Could you check a few things on this model? Use its own coordinates, in mm. Face numbers are marked on the shaded views. A direction names the side the tool comes from. Give positions to 0.01 mm unless a question says otherwise; leave off trailing zeros. Loops run counter-clockwise (first coordinate to the right, second up) from the corner with the lowest first, then second, coordinate; pieces in that order, holes last. Notation, with made-up numbers: M 76.5,52.25 L 96.5,52.25 A18 ccw 96.5,81.25 Z; hole C 17,57.5 d9. An arc over 180 degrees is marked long. Return JSON: item names as keys, results as strings. Group by question number.
1. If we section it at D-D (z = 0.25): Write out the boundary of the cut face in (x, y).
2. For the marked faces 1, 2 and 3, which set-ups out of +Z, -Z, +X, -X, +Y, -Y let a thin tool reach every point of the face, with its end or its side?
3. If we mould it in two halves opening along Y, with no side actions, what happens to the marked faces 4, 5 and 6? For each: +Y half, -Y half, draft (parallel to the pull), parting line (faces both ways), or undercut.
4. If we section it at B-B (z = -6.25): Write out the boundary of the cut face in (x, y), plus the area to 3 significant figures.
5. Please list where these lines run through material, in increasing order: line 1 (X direction, y = -124, z = 0.25); line 2 (X direction, y = -98.5, z = -7.35); line 3 (Y direction, x = 53, z = 0.6).
6. If we section it at A-A (y = -98.5): Write out the boundary of the cut face in (x, z), plus the area to 3 significant figures.
7. For pin 1 (4.5 mm diameter, centred on x = 53, y = -98.5, fed in from +Z); pin 2 (11.5 mm diameter, centred on x = 51.5, y = -96.5, fed in from +Z); pin 3 (5.5 mm diameter, centred on x = 53, y = -132, fed in from +Z); pin 4 (14.5 mm diameter, centred on x = 52, y = -126.5, fed in from -Z), each with a flat end and sliding along its axis, tell me the tip position at first contact or that it passes through.
8. If we section it at C-C (y = -124): Write out the boundary of the cut face in (x, z).
```python
from build123d import *

# Parameters (mm, degrees)
PAD024_DEPTH    = 13.5
SKETCH067_R     = 2.9
POCKET045_DEPTH = 5.001
SKETCH068_R     = 5.5
POCKET046_DEPTH = 3
SKETCH069_R     = 2.1
POCKET047_DEPTH = 7.001
CHAMFER023_SIZE = 4.99
FILLET014_R     = 10
CHAMFER024_SIZE = 3
CHAMFER025_SIZE = 0.2
CHAMFER026_SIZE = 1
CHAMFER027_SIZE = 1
CHAMFER028_SIZE = 0.4


with BuildPart() as part:
    # Sketch066 → Pad024 (new body, symmetric)
    with BuildSketch(Plane.YZ):
        Polygon((23, 0), (0, 0), (0, 7), (-28, 7), (-28, 0), (-10, 0), (-10, -5), (23, -5), align=None)
    extrude(amount=PAD024_DEPTH, both=True)

    # Sketch067 → Pocket045 (cut, through all)
    with BuildSketch(Plane.XY):
        with Locations((0, 11.5)):
            Circle(SKETCH067_R)
    extrude(amount=-POCKET045_DEPTH, mode=Mode.SUBTRACT)

    # Sketch068 (on Face7 of Pocket045) → Pocket046 (cut)
    with BuildSketch(Plane(origin=(0, 0, -5), x_dir=(1, 0, 0), z_dir=(0, 0, -1))):
        with Locations((0, -11.5)):
            Circle(SKETCH068_R)
    extrude(amount=-POCKET046_DEPTH, mode=Mode.SUBTRACT)

    # Sketch069 (on Face10 of Pocket046) → Pocket047 (cut, through all)
    with BuildSketch(Plane(origin=(0, 0, 0), x_dir=(1, 0, 0), z_dir=(0, 0, -1))):
        with Locations((0, 22)):
            Circle(SKETCH069_R)
        with Locations((-6, 14)):
            Circle(SKETCH069_R)
        with Locations((6, 14)):
            Circle(SKETCH069_R)
    extrude(amount=-POCKET047_DEPTH, mode=Mode.SUBTRACT)

    # Chamfer023
    chamfer023_edges = [part.edges().sort_by_distance(p)[0] for p in [
        (0, -10, -5),
    ]]
    chamfer(chamfer023_edges, length=CHAMFER023_SIZE)

    # Fillet014
    fillet014_edges = [part.edges().sort_by_distance(p)[0] for p in [
        (13.5, 23, -2.5),
        (-13.5, 23, -2.5),
    ]]
    fillet(fillet014_edges, radius=FILLET014_R)

    # Chamfer024
    chamfer024_edges = [part.edges().sort_by_distance(p)[0] for p in [
        (13.5, -28, 3.5),
        (-13.5, -28, 3.5),
    ]]
    chamfer(chamfer024_edges, length=CHAMFER024_SIZE)

    # Chamfer025
    chamfer025_edges = [part.edges().sort_by_distance(p)[0] for p in [
        (-2.9, 11.5, 0),
        (-2.9, 11.5, -2),
        (-5.5, 11.5, -5),
    ]]
    chamfer(chamfer025_edges, length=CHAMFER025_SIZE)

    # Chamfer026
    chamfer026_edges = [part.edges().sort_by_distance(p)[0] for p in [
        (3.9, -14, 0),
        (3.9, -14, 7),
        (-2.1, -22, 7),
        (-2.1, -22, 0),
        (-8.1, -14, 0),
        (-8.1, -14, 7),
    ]]
    chamfer(chamfer026_edges, length=CHAMFER026_SIZE)

    # Chamfer027
    chamfer027_edges = [part.edges().sort_by_distance(p)[0] for p in [
        (0, 0, 7),
    ]]
    chamfer(chamfer027_edges, length=CHAMFER027_SIZE)

    # Chamfer028
    chamfer028_edges = [part.edges().sort_by_distance(p)[0] for p in [
        (-13.5, -13, 7),
        (0, -1, 7),
        (-12, -26.5, 7),
        (13.5, -13, 7),
        (0, -28, 7),
        (12, -26.5, 7),
        (2.9, -14, 7),
        (-3.1, -22, 7),
        (-9.1, -14, 7),
    ]]
    chamfer(chamfer028_edges, length=CHAMFER028_SIZE)


with BuildPart() as part_1:
    # Body013 placement: moved
    add(part.part.moved(Location((53, -110, -3.7))))


solid = part_1.part
```
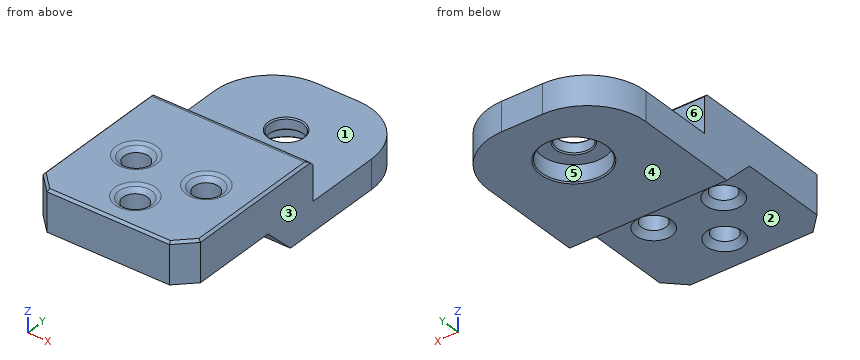
Answer:
{
 "1": {"outline": "M 39.5,-135 L 42.5,-138 L 63.5,-138 L 66.5,-135 L 66.5,-110 L 39.5,-110 Z; hole C 47,-124 d4.2; hole C 53,-132 d4.2; hole C 59,-124 d4.2"},
 "2": {"face 1": "+Z, +X, -X, +Y", "face 2": "-Z, +X, -X, -Y", "face 3": "+Z, -Z, +X, +Y, -Y"},
 "3": {"face 4": "draft", "face 5": "undercut", "face 6": "+Y half"},
 "4": {"outline": "M 39.5,-117.46 L 66.5,-117.46 L 66.5,-97 A10 ccw 56.5,-87 L 49.5,-87 A10 ccw 39.5,-97 Z; hole C 53,-98.5 d11", "area": "684 mm²"},
 "5": {"line 1": "x = 39.5 to 44.9, 49.1 to 56.9, 61.1 to 66.5", "line 2": "x = 39.5 to 47.5, 58.5 to 66.5", "line 3": "y = -138 to -134.1, -129.9 to -110"},
 "6": {"outline": "M 39.5,-8.7 L 47.3,-8.7 L 47.5,-8.5 L 47.5,-5.7 L 49.9,-5.7 L 50.1,-5.5 L 50.1,-3.9 L 49.9,-3.7 L 39.5,-3.7 Z; M 55.9,-5.5 L 56.1,-5.7 L 58.5,-5.7 L 58.5,-8.5 L 58.7,-8.7 L 66.5,-8.7 L 66.5,-3.7 L 56.1,-3.7 L 55.9,-3.9 Z", "area": "90.3 mm²"},
 "7": {"pin 1": "passes through", "pin 2": "stops at z = -3.7", "pin 3": "stops at z = 2.95", "pin 4": "stops at z = -4.46"},
 "8": {"outline": "M 39.5,-3.7 L 43.9,-3.7 L 44.9,-2.7 L 44.9,2.3 L 44.18,3.02 L 43.5,3.3 L 39.9,3.3 L 39.5,2.9 Z; M 49.1,-2.7 L 50.1,-3.7 L 55.9,-3.7 L 56.9,-2.7 L 56.9,2.3 L 56.18,3.02 L 55.5,3.3 L 50.5,3.3 L 49.82,3.02 L 49.1,2.3 Z; M 61.1,-2.7 L 62.1,-3.7 L 66.5,-3.7 L 66.5,2.9 L 66.1,3.3 L 62.5,3.3 L 61.82,3.02 L 61.1,2.3 Z"}
}
